Here's how the part is built. I have some questions about the finished solid (model axes, mm). Coordinates: 2 decimals unless noted, no trailing zeros. Loops run counter-clockwise (first coordinate to the right, second up) from the corner with the lowest first, then second, coordinate; pieces in that order, holes last. Notation, with made-up numbers: (57.5, 37) - (74.5, 37) arc R28 cw to (74.5, 73) - close; hole circle Ø7 at (77.5, -19). An arc over 180 degrees is marked (long way). Use a Markdown table: item, result.
Autodesk Inventor part; units mm, degrees
ref_plane "YZ Plane" through (0, 0, 0) normal (1, 0, 0) x (0, 1, 0)
ref_plane "XZ Plane" through (0, 0, 0) normal (0, 1, 0) x (-1, 0, 0)
ref_plane "XY Plane" through (0, 0, 0) normal (0, 0, 1) x (1, 0, 0)
sketch "Sketch1" plane through (0, 0, 0) normal (0, 0, 1) x (1, 0, 0)
  line L0 (-28.5, -28.5) -> (28.5, -28.5)
  line L1 (28.5, -28.5) -> (28.5, 28.5)
  line L2 (28.5, 28.5) -> (-28.5, 28.5)
  line L3 (-28.5, 28.5) -> (-28.5, -28.5)
  line L4 (-28.5, -28.5) -> (28.5, 28.5) construction
  line L5 (28.5, -28.5) -> (-28.5, 28.5) construction
  point P0 (0, 0)
  dimension "d0" = 57
  dimension "d1" = 57
extrude "Extrusion1" add sketch "Sketch1" against normal blind 2.921
sketch "Sketch2" plane through (0, 0, 0) normal (0, 0, 1) x (1, 0, 0)
  line L0 (-28.5, 28.5) -> (-9.5, 28.5)
  line L1 (-9.5, 28.5) -> (-9.5, 25.5)
  line L2 (-9.5, 25.5) -> (-25.5, 25.5)
  line L3 (-28.5, 22.4359) -> (-28.5, 28.5)
  line L4 (-28.5, 28.5) -> (-22.225, 28.5)
  line L5 (-25.5, 25.5) -> (-25.5, 9.5)
  line L6 (-25.5, 9.5) -> (-28.5, 9.5)
  line L7 (-28.5, 9.5) -> (-28.5, 28.5)
  line L8 (28.5, 28.5) -> (-28.5, 28.5)
  line L9 (-28.5, 28.5) -> (-28.5, -28.5)
  line L10 (0, 4.0972) -> (0, 8.5289)
  line L11 (-5.3828, 0) -> (-2.3228, 0)
  line L12 (28.5, 28.5) -> (9.5, 28.5)
  line L13 (9.5, 28.5) -> (9.5, 25.5)
  line L14 (9.5, 25.5) -> (25.5, 25.5)
  line L15 (28.5, 22.4359) -> (28.5, 28.5)
  line L16 (28.5, 28.5) -> (22.225, 28.5)
  line L17 (25.5, 25.5) -> (25.5, 9.5)
  line L18 (25.5, 9.5) -> (28.5, 9.5)
  line L19 (28.5, 9.5) -> (28.5, 28.5)
  line L20 (-28.5, -28.5) -> (-9.5, -28.5)
  line L21 (-9.5, -28.5) -> (-9.5, -25.5)
  line L22 (-9.5, -25.5) -> (-25.5, -25.5)
  line L23 (-28.5, -22.4359) -> (-28.5, -28.5)
  line L24 (-28.5, -28.5) -> (-22.225, -28.5)
  line L25 (-25.5, -25.5) -> (-25.5, -9.5)
  line L26 (-25.5, -9.5) -> (-28.5, -9.5)
  line L27 (-28.5, -9.5) -> (-28.5, -28.5)
  line L28 (28.5, -28.5) -> (-28.5, -28.5)
  line L29 (28.5, -28.5) -> (9.5, -28.5)
  line L30 (9.5, -28.5) -> (9.5, -25.5)
  line L31 (9.5, -25.5) -> (25.5, -25.5)
  line L32 (28.5, -22.4359) -> (28.5, -28.5)
  line L33 (28.5, -28.5) -> (22.225, -28.5)
  line L34 (25.5, -25.5) -> (25.5, -9.5)
  line L35 (25.5, -9.5) -> (28.5, -9.5)
  line L36 (28.5, -9.5) -> (28.5, -28.5)
  line L37 (-28.5, -28.5) -> (28.5, -28.5)
  line L38 (28.5, -28.5) -> (28.5, 28.5)
  point P0 (0, -8.5289)
  dimension "d59" = 3
  dimension "d62" = 3
  dimension "d65" = 19
  dimension "d66" = 19
  dimension "d67" = 19
  dimension "d68" = 19
  dimension "d69" = 19
  dimension "d70" = 19
  dimension "d71" = 19
  dimension "d72" = 19
  dimension "d73" = 19
  dimension "d74" = 19
  dimension "d75" = 19
  dimension "d76" = 19
extrude "Extrusion3" cut sketch "Sketch2" against normal up to next contours L0 L1 L2 L5 L6 L7 L3 | L8 L15 L19 L18 L17 L14 L13 | L26 L25 L22 L21 L20 L9 | L36 L32 L28 L30 L31 L34 L35
hole "Hole1" at (0, 0, 0) direction (0, 0, -1) diameter 25.4 end through all
equation "\"d1\" = d0"
equation "\"d62\" = d59"
equation "\"d68\" = d65"
equation "\"d70\" = d66"
equation "\"d23\" = 0.5 * d0"
equation "\"d53\" = 0.5 * d0"
properties part number "Top"
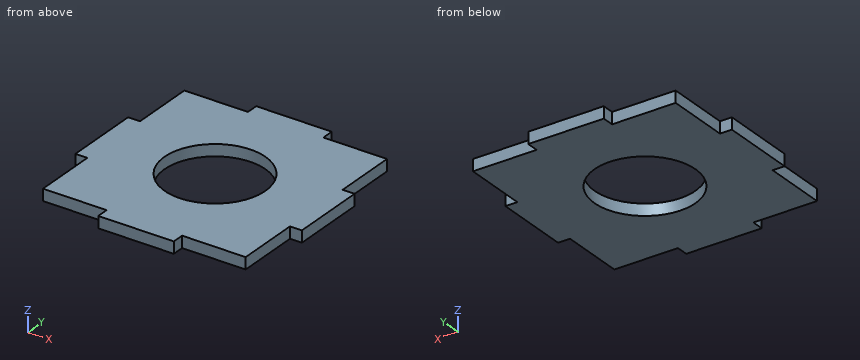
Q1. I want a section at D-D, the plane x = 17. Write out the boundary of the cut face in (y, z).
Check values:
| item | result |
|---|---|
| outline | (-25.5, -2.92) - (25.5, -2.92) - (25.5, 0) - (-25.5, 0) - close |
Q2. I want a section at A-A, the plane y = 0. Write out the boundary of the cut face in (x, z).
Check values:
| item | result |
|---|---|
| outline | (-28.5, -2.92) - (-12.7, -2.92) - (-12.7, 0) - (-28.5, 0) - close; (12.7, -2.92) - (28.5, -2.92) - (28.5, 0) - (12.7, 0) - close |
Q3. I want a section at C-C, the plane z = -1.6. Write out the boundary of the cut face in (x, y).
Check values:
| item | result |
|---|---|
| outline | (-28.5, -9.5) - (-25.5, -9.5) - (-25.5, -25.5) - (-9.5, -25.5) - (-9.5, -28.5) - (9.5, -28.5) - (9.5, -25.5) - (25.5, -25.5) - (25.5, -9.5) - (28.5, -9.5) - (28.5, 9.5) - (25.5, 9.5) - (25.5, 25.5) - (9.5, 25.5) - (9.5, 28.5) - (-9.5, 28.5) - (-9.5, 25.5) - (-25.5, 25.5) - (-25.5, 9.5) - (-28.5, 9.5) - close; hole circle Ø25.4 at (0, 0) |
Q4. Please list where these lines run through material, in increasing order: L1, parallel to Y at x = 0, z = -1.7; L2, parallel to X at y = 23, z = -1.95. Write a range as from..to.
Check values:
| item | result |
|---|---|
| L1 | -28.5..-12.7, 12.7..28.5 |
| L2 | -25.5..25.5 |
Q5. Will these pins go through, and if not, where does the flat tip stop? P1, Ø1.5, axis at y = -14.5, z = -1.5, coming from the -X side; P2, Ø1.5, axis at x = 14.5, z = -1.5, coming from the +Y side; P3, Ø0.9, axis at y = -26.5, z = -1, coming from the -X side.
Check values:
| item | result |
|---|---|
| P1 | x = -25.5 |
| P2 | y = 25.5 |
| P3 | x = -9.5 |
